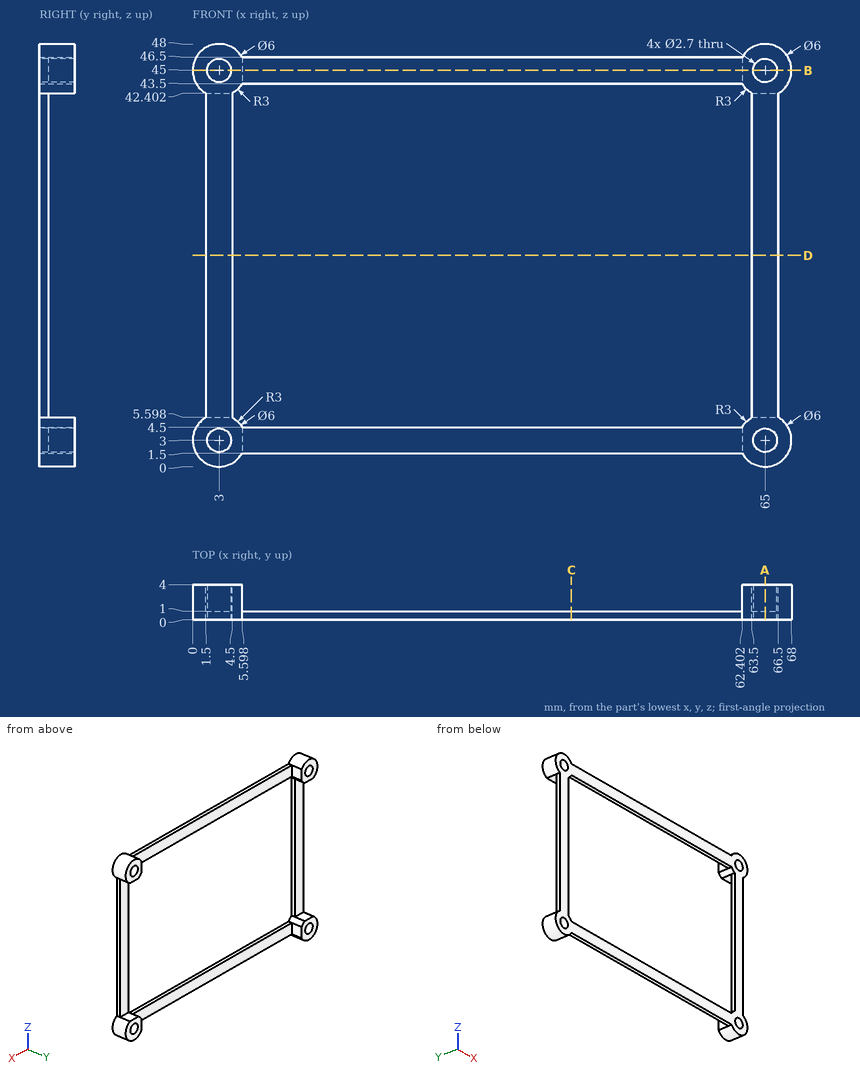
Geometry: see drawing. Coordinates: mm, zero at the bounding-box minimum. Round coordinates to 2 decimals unless told otherwise and drop trailing zeros. Order: outer loops, then holes, each group sorted by start corner. A loop starts at its lowest first (then second) coordinate and runs counter-clockwise, first axis right, second up. Notation, with made-up numbers: (41.25, -30) - (48.25, -30) arc R27 cw to (48.25, 9) - close; hole circle Ø5 at (-0.75, 28.25). An arc over 180 degrees is marked (long way). Use a Markdown table: item, result. Add a question column.
1. Section query A-A (x = 65). Return the cut outline in (y, z), then the cut area to 3 significant figures.
2. Line query: probe 1 along Z at (x, y) = (65, 1.3); probe 2 along Z at (x, y) = (46, 0.8); probe 3 along X at (y, z) = (0.45, 20). Output: solid intervals per line, ascending.
3. Section query B-B (z = 45). Return the cut outline in (x, y).
4. Section query C-C (x = 43). Return the cut outline in (y, z).
5. Section query D-D (z = 24). Return the cut outline in (x, y), then the cut area to 3 significant figures.
6. First-contact query: pin 1 (2.5 mm diameter, centred on x = 3.5, z = 28, fed in from +Y); pin 2 (0.8 mm diameter, centred on y = 0.5, z = 16, fed in from +X); pin 3 (0.5 mm diameter, centred on x = 33, y = 0.5, fed in from -Z). Flat tips, straight axial feed; report the tip coordinate or a pass-through.
Derived:
| question | item | result |
|---|---|---|
| 1 | outline | (0, 0) - (4, 0) - (4, 1.65) - (0, 1.65) - close; (0, 4.35) - (4, 4.35) - (4, 5.6) - (1, 5.6) - (1, 42.4) - (4, 42.4) - (4, 43.65) - (0, 43.65) - close; (0, 46.35) - (4, 46.35) - (4, 48) - (0, 48) - close |
| 1 | area | 60.0 mm2 |
| 2 | probe 1 | 0 to 1.65, 4.35 to 5.6, 42.4 to 43.65, 46.35 to 48 |
| 2 | probe 2 | 1.5 to 4.5, 43.5 to 46.5 |
| 2 | probe 3 | 1.5 to 4.5, 63.5 to 66.5 |
| 3 | outline | (0, 0) - (1.65, 0) - (1.65, 4) - (0, 4) - close; (4.35, 0) - (63.65, 0) - (63.65, 4) - (62.4, 4) - (62.4, 1) - (5.6, 1) - (5.6, 4) - (4.35, 4) - close; (66.35, 0) - (68, 0) - (68, 4) - (66.35, 4) - close |
| 4 | outline | (0, 1.5) - (1, 1.5) - (1, 4.5) - (0, 4.5) - close; (0, 43.5) - (1, 43.5) - (1, 46.5) - (0, 46.5) - close |
| 5 | outline | (1.5, 0) - (4.5, 0) - (4.5, 1) - (1.5, 1) - close; (63.5, 0) - (66.5, 0) - (66.5, 1) - (63.5, 1) - close |
| 5 | area | 6.00 mm2 |
| 6 | pin 1 | y = 1 |
| 6 | pin 2 | x = 66.5 |
| 6 | pin 3 | z = 1.5 |
